Model file for the job. Use its own axes, mm. A direction names the side the tool comes from. Round coordinates to 2 decimals unless told otherwise and drop trailing zeros. Loops run counter-clockwise (first coordinate to the right, second up) from the corner with the lowest first, then second, coordinate; pieces in that order, holes last. Notation, with made-up numbers: M 43,-28 L 98,-28 A10 cw 98,-18 Z; hole C -4,-0.75 d9. An arc over 180 degrees is marked long. Use a Markdown table: item, result. Add a question column.
Q1. Cut at D-D (x = 201.5). Give the cut face in (y, z) (3 decimals).
Q2. Cut at A-A (x = 78.5). Give the cut face in (y, z) (3 decimals).
Q3. Probe line 1 (Z direction, x = 141, y = 2) (3 decimals); line 2 (X direction, y = 6.35, z = 20.6); line 3 (Y direction, x = 209.5, z = -12) (3 decimals). List the from-to ranges inside material, lowest first. Write a range as from..to.
Q4. Pin check, flat tip, straight feed: pin 1 (8 mm diameter, centred on x = 19.05, y = 32.385, fed in from -Z). Stop position of the tip, or through.
Q5. Tool access for faces 1 (the face through (24.1, 20.35, -20.62)), 2 (the face through (116, 19, 22.225)), 3 (the face through (116, 0, -4)): list every direction of +Z, -Z, +X, -X, +Y, -Y with a clear straight run to the whole face (end or side of a thin tool).
Q6. Cut at B-B (z = 0). Give the cut face in (x, y) (3 decimals).
Q7. Cut at C-C (y = 23). Give the cut face in (x, z) (3 decimals), plus the area to 3 significant figures.
Q8. Mould opens along Z. For faces 4 (the face through (231.43, 5.8, 20.66)), 5 (the face through (116, 20, 19.05)), 6 (the face through (116, 19, -22.225)) say: +Z half, -Z half, draft (parallel to the pull), parting line (faces both ways), or undercut.
Autodesk Inventor part; units mm, degrees
ref_plane "YZ Plane" through (0, 0, 0) normal (1, 0, 0) x (0, 1, 0)
ref_plane "XZ Plane" through (0, 0, 0) normal (0, 1, 0) x (-1, 0, 0)
ref_plane "XY Plane" through (0, 0, 0) normal (0, 0, 1) x (1, 0, 0)
sketch "Sketch1" plane through (0, 0, 0) normal (1, 0, 0) x (0, 1, 0)
  line L0 (41.275, -22.225) -> (-3.175, -22.225)
  line L1 (-3.175, -22.225) -> (-3.175, 22.225)
  line L2 (-3.175, 22.225) -> (41.275, 22.225)
  line L3 (0, 19.05) -> (0, -19.05)
  line L4 (0, 19.05) -> (41.275, 19.05)
  line L5 (0, -19.05) -> (41.275, -19.05)
  line L6 (41.275, 22.225) -> (41.275, 19.05)
  line L7 (41.275, -19.05) -> (41.275, -22.225)
  point P0 (0, 0)
  point P1 (0, 0)
  dimension "d27" = 44.45
  dimension "d28" = 44.45
  dimension "d29" = 3.175
  dimension "d83" = 3.175
extrude "Extrusion1" add sketch "Sketch1" along normal blind 236.1946
sketch "Sketch4" plane through (0, -3.175, -22.225) normal (0, 0, -1) x (-1, 0, 0)
  line L0 (0, 3.175) -> (0, 0)
  line L1 (-44.45, 101.8817) -> (-44.45, -23.3371)
  line L2 (0, 3.175) -> (-236.1946, 3.175)
  point P0 (-19.05, 35.56)
  point P1 (-69.85, 35.56)
  dimension "d30" = 50.8
  dimension "d81" = 25.4
  dimension "d82" = 44.45
  dimension "d84" = 32.385
hole "Hole2" at (19.05, 32.385, -22.225) at (69.85, 32.385, -22.225) direction (0, 0, 1) diameter 5.1054 end through all
sketch "Sketch7" plane through (0, -3.175, 0) normal (0, 0, 1) x (1, 0, 0)
  line L0 (-1.0792, 48.7042) -> (44.45, 94.2334)
  line L1 (44.45, 94.2334) -> (89.9792, 48.7042)
  line L2 (89.9792, 48.7042) -> (44.45, 3.175)
  line L3 (44.45, 3.175) -> (-1.0792, 48.7042)
  line L4 (0, 0) -> (0, 44.45)
  line L5 (0, 0) -> (236.1946, 0)
  line L6 (44.45, 3.175) -> (44.45, -64.4339)
  circle A0 centre (19.05, 35.56) radius 2.5527
  circle A1 centre (69.85, 35.56) radius 2.5527
  point P0 (0, 3.175)
  dimension "d57" = 3.175
  dimension "d85" = 50.8
  dimension "d86" = 25.4
  dimension "d87" = 135
extrude "Extrusion3" cut sketch "Sketch7" against normal through all contours L0 L1 L2 L3 | A0 | A1
sketch "Sketch10" plane through (0, -3.175, 0) normal (0, 0, 1) x (1, 0, 0)
  line L0 (31.75, 54.9704) -> (57.15, 54.9704)
  line L1 (57.15, 54.9704) -> (57.15, 35.56)
  line L2 (31.75, 35.56) -> (31.75, 54.9704)
  arc A0 (31.75, 35.56) -> (57.15, 35.56) centre (44.45, 35.56) ccw
  circle A1 centre (19.05, 35.56) radius 2.5527
  point P0 (0, 3.175)
  point P1 (44.45, 3.175)
  dimension "d88" = 25.4
extrude "Extrusion5" cut sketch "Sketch10" along normal through all contours L0 L1 A0 L2
sketch "Sketch11" plane through (0, -3.175, -22.225) normal (0, 0, -1) x (-1, 0, 0)
  line L0 (-236.1946, 0) -> (-236.1946, 44.45)
  line L1 (0, 0) -> (-236.1946, 0)
  arc A0 (-57.15, 35.56) -> (-31.75, 35.56) centre (-44.45, 35.56) ccw
  line L2 (-85.725, 44.45) -> (-236.1946, 44.45)
  point P0 (0, 3.175)
  point P1 (-203.537, 18.542)
  point P2 (-236.1946, 22.225)
  dimension "d89" = 159.9946
  dimension "d114" = 25.908
hole "Hole5" at (203.537, 15.367, -22.225) direction (0, 0, 1) diameter 28.5496 end through all
sketch "Sketch12" plane through (0, -3.175, -22.225) normal (0, 0, -1) x (-1, 0, 0)
  circle A0 centre (-203.537, 18.542) radius 14.2748
  line L0 (0, 0) -> (-236.1946, 0)
  point P0 (0, 3.175)
  point P1 (-178.137, 38.1)
  point P2 (-178.137, 9.525)
  point P3 (-228.937, 9.525)
  point P4 (-228.937, 38.1)
  dimension "d99" = 9.525
  dimension "d100" = 38.1
  dimension "d101" = 25.4
  dimension "d102" = 25.4
hole "Hole6" at (178.137, 34.925, -22.225) at (178.137, 6.35, -22.225) at (228.937, 6.35, -22.225) at (228.937, 34.925, -22.225) direction (0, 0, 1) diameter 5.1054 end through all
sketch "Sketch8" plane through (0, 0, 19.05) normal (0, 1, 0) x (1, 0, 0)
  line L0 (64.7446, 19.05) -> (90.1446, 19.05) construction
  line L1 (64.7446, 15.494) -> (90.1446, 15.494)
  line L2 (90.1446, 22.606) -> (64.7446, 22.606)
  arc A0 (64.7446, 22.606) -> (64.7446, 15.494) centre (64.7446, 19.05) ccw
  arc A1 (90.1446, 15.494) -> (90.1446, 22.606) centre (90.1446, 19.05) ccw
  line L3 (115.5446, 19.05) -> (140.9446, 19.05) construction
  line L4 (115.5446, 15.494) -> (140.9446, 15.494)
  line L5 (140.9446, 22.606) -> (115.5446, 22.606)
  arc A2 (115.5446, 22.606) -> (115.5446, 15.494) centre (115.5446, 19.05) ccw
  arc A3 (140.9446, 15.494) -> (140.9446, 22.606) centre (140.9446, 19.05) ccw
  line L6 (236.1946, 38.1) -> (236.1946, 0)
  line L7 (0, 0) -> (0, 38.1)
  point P0 (77.4446, 19.05)
  point P1 (128.2446, 19.05)
  point P2 (0, 19.05)
  dimension "d62" = 25.4
  dimension "d64" = 107.95
  dimension "d80" = 158.75
  dimension "d115" = 7.112
extrude "Extrusion4" cut sketch "Sketch8" against normal through all
ref_plane "Work Plane1" through (0, -3.175, 0) normal (0, 0, 1) x (1, 0, 0)
sketch "Sketch2" plane through (0, 0, 0) normal (0, 0, 1) x (1, 0, 0)
  circle A0 centre (23.8125, 23.8125) radius 25.4
  line L0 (5.852, 64.6197) -> (5.852, -28.4292) construction
  line L1 (0, 50.8) -> (0, 0) construction
  line L2 (0, 0) -> (304.8, 0) construction
  line L3 (304.8, 50.8) -> (304.8, 0) construction
  line L4 (0, 50.8) -> (304.8, 50.8) construction
  line L5 (0, 47.625) -> (304.8, 47.625) construction
  point P0 (5.852, 5.852)
  point P1 (41.773, 5.852)
  point P2 (41.773, 41.773)
  point P3 (5.852, 41.773)
  dimension "d11" = 50.8
  dimension "d14" = 360
  dimension "d16" = 5.852
  dimension "d17" = 5.852
  dimension "d19" = 5.852
equation "\"d83\" = d29"
equation "\"d86\" = 0.5 * d85"
equation "\"d19\" = d17"
properties part number "CAR_042_KickerLBracket" material "Aluminum 6061"
Checked values:
| question | item | result |
|---|---|---|
| 1 | outline | M -3.175,-22.225 L 1.238,-22.225 L 1.238,-19.05 L 0,-19.05 L 0,19.05 L 1.238,19.05 L 1.238,22.225 L -3.175,22.225 Z; M 29.496,-22.225 L 41.275,-22.225 L 41.275,-19.05 L 29.496,-19.05 Z; M 29.496,19.05 L 41.275,19.05 L 41.275,22.225 L 29.496,22.225 Z |
| 2 | outline | M -3.175,-22.225 L 34.05,-22.225 L 34.05,-19.05 L 0,-19.05 L 0,-3.556 L -3.175,-3.556 Z; M -3.175,3.556 L 0,3.556 L 0,19.05 L 41.275,19.05 L 41.275,22.225 L -3.175,22.225 Z |
| 3 | line 1 | z = -22.225..-19.05, 19.05..22.225 |
| 3 | line 2 | x = 0..175.58, 180.69..192.47, 214.6..226.38, 231.49..236.19 |
| 3 | line 3 | y = -3.175..0 |
| 4 | pin 1 | stops at z = 19.05 |
| 5 | face 1 | -Z, +Y |
| 5 | face 2 | +Z, +X, -X, +Y, -Y |
| 5 | face 3 | +X, -X, +Y |
| 6 | outline | M 0,-3.175 L 61.189,-3.175 L 61.189,0 L 0,0 Z; M 93.701,-3.175 L 111.989,-3.175 L 111.989,0 L 93.701,0 Z; M 144.501,-3.175 L 236.195,-3.175 L 236.195,0 L 144.501,0 Z |
| 7 | outline | M 0,-22.225 L 21.45,-22.225 L 21.45,-19.05 L 0,-19.05 Z; M 0,19.05 L 35.894,19.05 L 35.894,22.225 L 0,22.225 Z; M 53.006,19.05 L 191.474,19.05 L 191.474,22.225 L 53.006,22.225 Z; M 67.45,-22.225 L 191.474,-22.225 L 191.474,-19.05 L 67.45,-19.05 Z; M 215.6,-22.225 L 236.195,-22.225 L 236.195,-19.05 L 215.6,-19.05 Z; M 215.6,19.05 L 236.195,19.05 L 236.195,22.225 L 215.6,22.225 Z |
| 7 | area | 1,150 mm^2 |
| 8 | face 4 | draft |
| 8 | face 5 | undercut |
| 8 | face 6 | -Z half |
